Geometry: see drawing. Coordinates: mm, zero at the bounding-box minimum. A direction names the side the tool comes from. Round coordinates to 2 decimals unless told otherwise and drop trailing zeros. Loops run counter-clockwise (first coordinate to the right, second up) from the corner with the lowest first, then second, coordinate; pieces in that order, holes last. Notation, with made-up numbers: (52, -26) - (92, -26) arc R19 cw to (92, 1) - close; hole circle Ø11 at (52.5, -24). An arc over 180 degrees is marked (long way). Use CSV: the item, a comma, the result in double quotes. Start each with the question number.
1. Access query for the marked faces 1 and 2. Directions: +Z, -Z, +X, -X, +Y, -Y. A direction counts if a zero-diameter tool reaches every point of the face in a straight line with its end or side. Return the directions, or none.
2. Pin query (flat end, axial travel): P1, Ø1.5, axis at y = 37.5, z = 17.5, coming from the -X side (1 decimal); P2, Ø11, axis at x = 33.5, z = 38, coming from the -Y side; P3, Ø6, axis at y = 62, z = 65.5, coming from the -X side (1 decimal). Return the tip coordinate at first contact, or that it passes through.
3. Cut plane C-C (z = 39.5). Return loops of the section in (x, y), and give its area (3 significant figures).
4. Cut plane A-A (x = 37.5). Return loops of the section in (y, z).
5. Cut plane B-B (y = 75). Return loops of the section in (x, z).
6. Material intervals for probe 1 along Y at (x, z) = (37, 114) (1 decimal); probe 2 along Z at (x, y) = (61, 48); probe 3 along X at (y, z) = (42.5, 71), sorted ascending. Write a range as from..to.
7. Cut plane D-D (z = 63.5). Return loops of the section in (x, y), and give its area (3 significant figures).
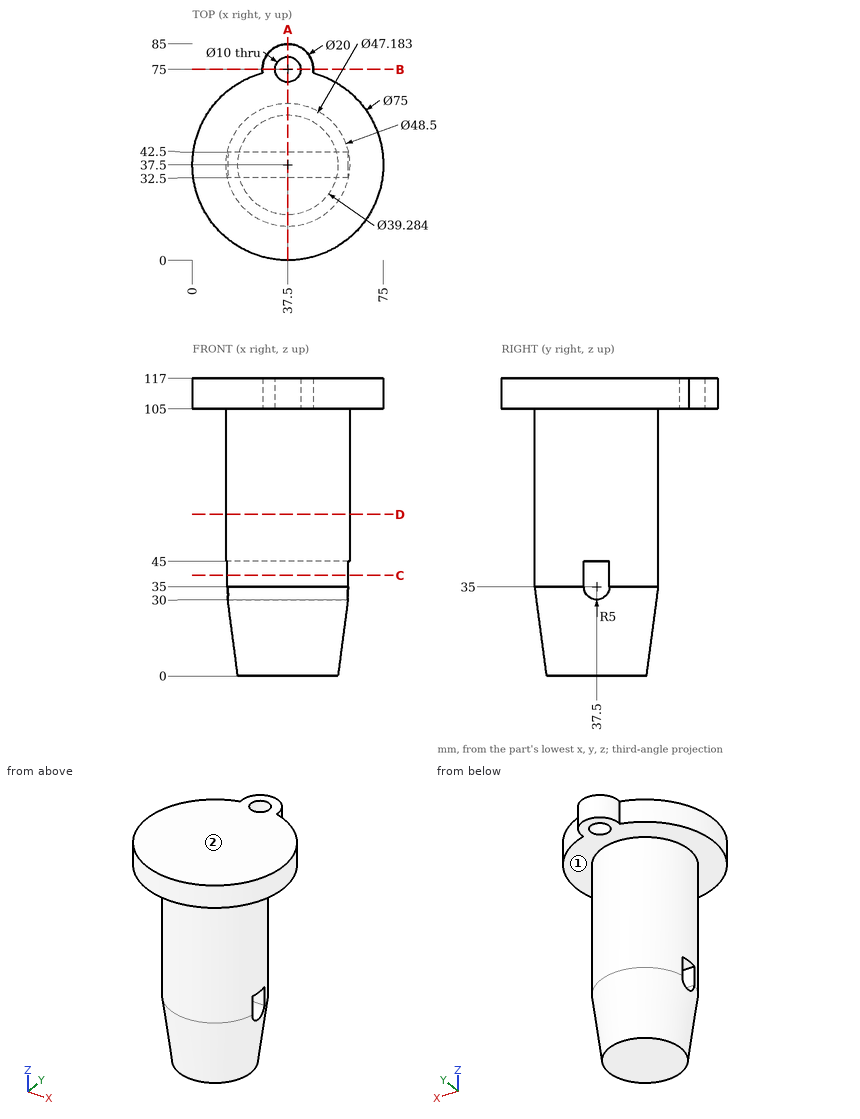
Established:
1,face 1,"-Z"
1,face 2,"+Z, +X, -X, +Y, -Y"
2,P1,"stops at x = 15.5"
2,P2,"stops at y = 13.25"
2,P3,"stops at x = 26.3"
3,outline,"(13.77, 32.5) arc R24.25 ccw to (61.23, 32.5) - close; (13.77, 42.5) - (61.23, 42.5) arc R24.25 ccw to start"
3,area,"1,370 mm2"
4,outline,"(0, 105) - (13.25, 105) - (13.25, 35) - (17.86, 0) - (57.14, 0) - (61.75, 35) - (61.75, 105) - (70, 105) - (70, 117) - (0, 117) - close; (80, 105) - (85, 105) - (85, 117) - (80, 117) - close; hole (32.5, 35) arc R5 ccw to (42.5, 35) - (42.5, 45) - (32.5, 45) - close"
5,outline,"(27.5, 105) - (32.5, 105) - (32.5, 117) - (27.5, 117) - close; (42.5, 105) - (47.5, 105) - (47.5, 117) - (42.5, 117) - close"
6,probe 1,"y = 0..70, 80..85"
6,probe 2,"z = 105..117"
6,probe 3,"x = 13.77..61.23"
7,outline,"circle Ø48.5 at (37.5, 37.5)"
7,area,"1,850 mm2"
